Could you check a few things on this drawing? It's one solid part, dimensions in mm from its lowest x, y, z. Round coordinates to 2 decimals unless told otherwise and drop trailing zeros. Order: outer loops, then holes, each group sorted by start corner. A loop starts at its lowest first (then second) coordinate and runs counter-clockwise, first axis right, second up. Notation, with made-up numbers: (-12.75, 34) - (-2.75, 34) arc R25 ccw to (-2.75, 69) - close; hole circle Ø2 at (9, -4.75). An arc over 180 degrees is marked (long way). Use one line per item in the form item = value.
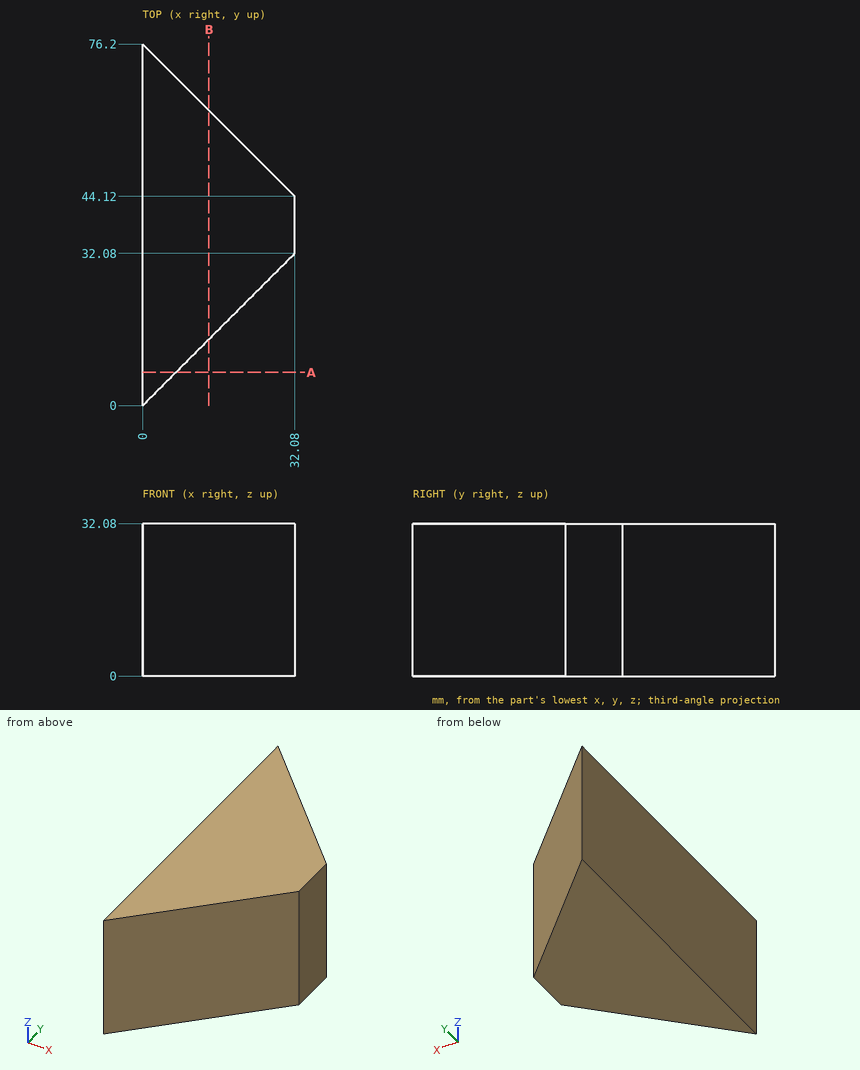
Item 1: I need wall thicknesses on L1, parallel to X at y = 63, z = 7; L2, parallel to Y at x = 16, z = 7.5; L3, parallel to Y at x = 27, z = 3. Which ranges of each line are inside material? Lowest first, please.
Found:
L1 = 0 to 13.2
L2 = 16 to 60.2
L3 = 27 to 49.2
Item 2: Imagine slicing it at A-A on y = 7. Please give me the cut outline in (x, z), plus the area to 3 significant figures.
Found:
outline = (0, 0) - (7, 0) - (7, 32.08) - (0, 32.08) - close
area = 225 mm2
Item 3: Imagine slicing it at B-B on x = 14. Please give me the cut outline in (y, z).
Found:
outline = (14, 0) - (62.2, 0) - (62.2, 32.08) - (14, 32.08) - close
Item 4: Will these pins go through, and if not, where does the flat tip stop? P1, Ø12, axis at y = 14.5, z = 20, coming from the +X side; P2, Ø3, axis at x = 23.5, z = 19, coming from the -Y side; P3, Ø5, axis at x = 21, z = 11, coming from the -Y side.
Found:
P1 = 20.5
P2 = 22
P3 = 18.5
